from build123d import *

# Parameters (mm, degrees)
EXTRUDE_5_DEPTH = 2
EXTRUDE_START   = -2
SKETCH_1_7_R    = 1.6
EXTRUDE_6_DEPTH = 2


with BuildPart() as part:
    # Sketch 1 → Extrude 5 (new body)
    with BuildSketch(Plane(origin=(0, 0, 0), x_dir=(1, 0, 0), z_dir=(0, 1, 0))):
        with BuildLine():
            ThreePointArc((-6.42, -8.22), (-7.692792206, -7.692792206), (-8.22, -6.42))
            Line((-8.22, -6.42), (-8.22, 6.42))
            ThreePointArc((-8.22, 6.42), (-7.692792206, 7.692792206), (-6.42, 8.22))
            Line((-6.42, 8.22), (6.42, 8.22))
            ThreePointArc((6.42, 8.22), (7.692792206, 7.692792206), (8.22, 6.42))
            Line((8.22, 6.42), (8.22, -6.42))
            ThreePointArc((8.22, -6.42), (7.692792206, -7.692792206), (6.42, -8.22))
            Line((6.42, -8.22), (-6.42, -8.22))
        make_face()
        Polygon((-2.85, -1.645448267), (0, -3.290896534), (2.85, -1.645448267), (2.85, 1.645448267), (0, 3.290896534), (-2.85, 1.645448267), align=None, mode=Mode.SUBTRACT)
    extrude(amount=EXTRUDE_5_DEPTH)

    # Sketch 1_7 → Extrude 6 (add)
    # profile 1 of 2: a face of its own
    with BuildSketch(Plane(origin=(0, 0, 0), x_dir=(1, 0, 0), z_dir=(0, 1, 0)).offset(EXTRUDE_START)):
        with BuildLine():
            ThreePointArc((-6.42, -8.22), (-7.692792206, -7.692792206), (-8.22, -6.42))
            Line((-8.22, -6.42), (-8.22, 6.42))
            ThreePointArc((-8.22, 6.42), (-7.692792206, 7.692792206), (-6.42, 8.22))
            Line((-6.42, 8.22), (6.42, 8.22))
            ThreePointArc((6.42, 8.22), (7.692792206, 7.692792206), (8.22, 6.42))
            Line((8.22, 6.42), (8.22, -6.42))
            ThreePointArc((8.22, -6.42), (7.692792206, -7.692792206), (6.42, -8.22))
            Line((6.42, -8.22), (-6.42, -8.22))
        make_face()
        Polygon((-2.85, -1.645448267), (0, -3.290896534), (2.85, -1.645448267), (2.85, 1.645448267), (0, 3.290896534), (-2.85, 1.645448267), align=None, mode=Mode.SUBTRACT)
    # profile 2 of 2: a face of its own
    with BuildSketch(Plane(origin=(0, 0, 0), x_dir=(1, 0, 0), z_dir=(0, 1, 0)).offset(EXTRUDE_START)):
        Polygon((-2.85, 1.645448267), (-2.85, -1.645448267), (0, -3.290896534), (2.85, -1.645448267), (2.85, 1.645448267), (0, 3.290896534), align=None)
        with Locations(Location((0, 0, 0), (0, 0, 270))):
            Circle(SKETCH_1_7_R, mode=Mode.SUBTRACT)
    extrude(amount=EXTRUDE_6_DEPTH)


solid = part.part
Model file for the job. Use its own axes, mm. A direction names the side the tool comes from. Round coordinates to 2 decimals unless told otherwise and drop trailing zeros. Order: outer loops, then holes, each group sorted by start corner. A loop starts at its lowest first (then second) coordinate and runs counter-clockwise, first axis right, second up. Notation, with made-up numbers: M 56.5,4.25 L 61.5,4.25 A28 cw 61.5,43.25 Z; hole C 15.5,-22 d1. An arc over 180 degrees is marked long. Write each question's results on one line, items separated by ' | '. Start each with the question number.
(1) Saw through at A-A, the plane z = 0. Give the cut face in (x, y).
(2) Which spindle directions (+Z, -Z, +X, -X, +Y, -Y) get a long thin tool onto all of the face, cutting with end or side? Do faces 1 (the face through (1.405, 0.986, 2.48)), 2 (the face through (4, 2, 0)). Say none if no direction does.
(3) Saw through at D-D, the plane z = 2.5. Give the cut face in (x, y), then the cut area to 3 significant figures.
(4) Saw through at B-B, the plane y = -0.2. Give the cut face in (x, z), then the cut area to 3 significant figures.
(5) Saw through at C-C, the plane y = 1.5. Give the cut face in (x, z), then the cut area to 3 significant figures.
(6) Drop flat-ended pins along their axis: pin 1 (1.9 mm diameter, centred on x = 0, z = 0, fed in from -Y); pin 2 (4.5 mm diameter, centred on x = 0, z = 0.5, fed in from +Y). Give the stop position or say it passes through.
(7) Probe probe 1 along X at (y, z) = (-0.7, 0.5); probe 2 along Z at (x, y) = (7.25, 0.8); probe 3 along X at (y, z) = (-1.45, -6.75). List the from-to ranges inside material, lowest first. Write a range as from..to.
(8) Two-plate mould, pull along X, no slides. Class faces 3 (the face through (-7.707, -0.028, -7.679)), 4 (the face through (0, 0, 8.22)), 5 (the face through (-1.44, 0.99, 2.46)): pulls with the +X half, pulls with the -X half, needs draft (parallel to the pull), parting line crosses it, or undercut.
Established:
1) outline: M -8.22,-2 L -1.6,-2 L -1.6,0 L -2.85,0 L -2.85,2 L -8.22,2 Z; M 1.6,-2 L 8.22,-2 L 8.22,2 L 2.85,2 L 2.85,0 L 1.6,0 Z
2) face 1: +Y | face 2: +Z, -Z, +X, -X, +Y
3) outline: M -8.22,-2 L 8.22,-2 L 8.22,2 L 1.37,2 L 1.37,0 L -1.37,0 L -1.37,2 L -8.22,2 Z | area: 60.3 mm^2
4) outline: M -8.22,-6.42 A1.8 ccw -6.42,-8.22 L 6.42,-8.22 A1.8 ccw 8.22,-6.42 L 8.22,6.42 A1.8 ccw 6.42,8.22 L -6.42,8.22 A1.8 ccw -8.22,6.42 Z; hole C 0,0 d3.2 | area: 259 mm^2
5) outline: M -8.22,-6.42 A1.8 ccw -6.42,-8.22 L 6.42,-8.22 A1.8 ccw 8.22,-6.42 L 8.22,6.42 A1.8 ccw 6.42,8.22 L -6.42,8.22 A1.8 ccw -8.22,6.42 Z; hole M -2.85,-1.65 L 0,-3.29 L 2.85,-1.65 L 2.85,1.65 L 0,3.29 L -2.85,1.65 Z | area: 239 mm^2
6) pin 1: passes through | pin 2: stops at y = 0
7) probe 1: x = -8.22..-1.52, 1.52..8.22 | probe 2: z = -8.02..8.02 | probe 3: x = -8.19..8.19
8) face 3: pulls with the -X half | face 4: needs draft | face 5: undercut
